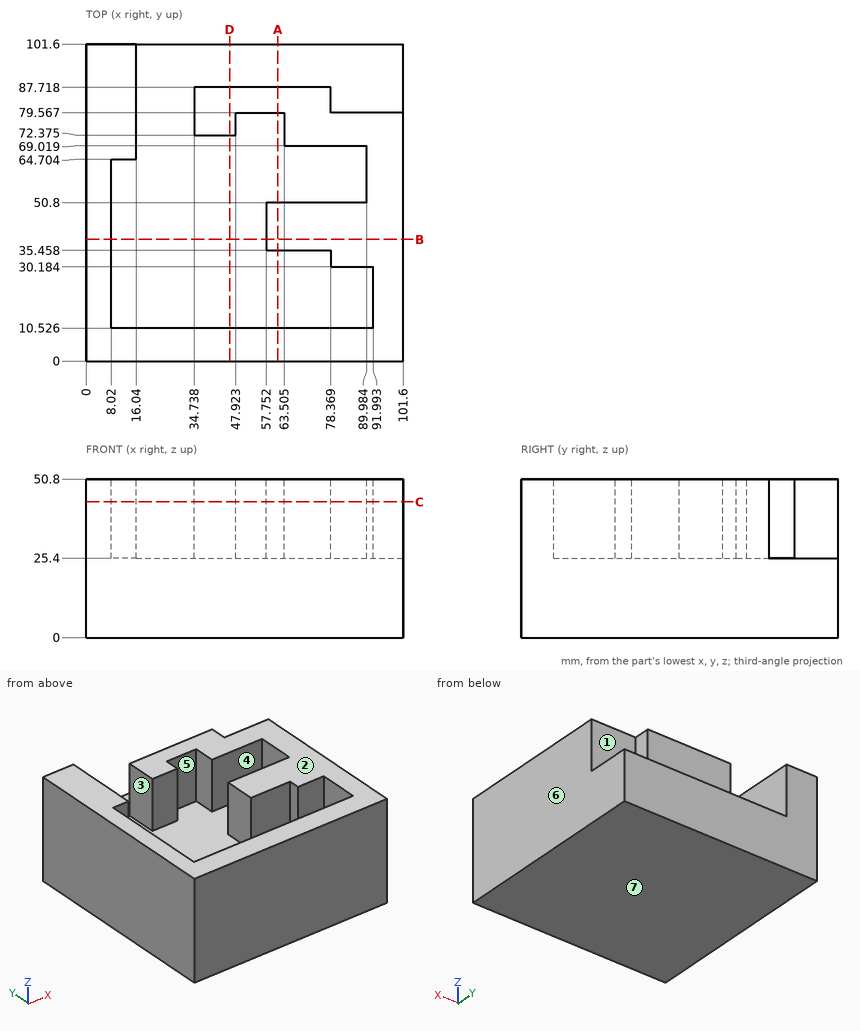
Geometry check sheet. Reference: drawing and pictorial views, mm from the part's lowest x, y, z. A direction names the side the tool comes from. Round coordinates to 2 decimals unless told otherwise and drop trailing zeros. Write each loop counter-clockwise with the first axis right and the second up, starting at its lowest first coordinate (ties: lowest second). Pieces come first, ordered by that corner, then holes.
(1) Depth check by flat-ended pin: pin 1 Ø6 at (x, y) = (20, 75.5) entering from +Z; pin 2 Ø6 at (x, z) = (85.5, 42.5) entering from +Y; pin 3 Ø6 at (x, z) = (71, 37.5) entering from +Y. Enter the tip coordinate at first touch or a pass-through.
Returned:
pin 1: stops at z = 25.4
pin 2: stops at y = 79.57
pin 3: stops at y = 87.72
(2) Section check B-B (y = 39). Enter the section's corners in (x, z).
Returned:
outline: (0, 0) - (101.6, 0) - (101.6, 50.8) - (57.75, 50.8) - (57.75, 25.4) - (8.02, 25.4) - (8.02, 50.8) - (0, 50.8) - close
(3) Material ranges on line 1 (X direction, y = 64, z = 39) (1 decimal); line 2 (Y direction, x = 42.5, z = 47.5) (1 decimal); line 3 (Y direction, x = 50.5, z = 40) (1 decimal), recorded low to high.
Returned:
line 1: x = 0 to 8, 90 to 101.6
line 2: y = 0 to 10.5, 72.4 to 87.7
line 3: y = 0 to 10.5, 79.6 to 87.7
(4) Section check A-A (x = 61.5). Enter the section's corners in (y, z) (1 decimal).
Returned:
outline: (0, 0) - (101.6, 0) - (101.6, 25.4) - (87.7, 25.4) - (87.7, 50.8) - (79.6, 50.8) - (79.6, 25.4) - (50.8, 25.4) - (50.8, 50.8) - (35.5, 50.8) - (35.5, 25.4) - (10.5, 25.4) - (10.5, 50.8) - (0, 50.8) - close
(5) Access from +Z, -Z, +X, -X, +Y, -Y to the whole of each face (thin tool, end or side, straight path). Record for the marked faces 1, 2, 3 and 4.
Returned:
face 1: +Z, +X, +Y
face 2: +Z, +X, -X, +Y, -Y
face 3: +Z, +Y
face 4: +Z
(6) Mould release check, pull along X, two halves, no side actions. Record for the marked faces 5, 6 and 7: pulls with the +X half, pulls with the -X half, needs draft (parallel to the pull), parting line crosses it, or undercut.
Returned:
face 5: undercut
face 6: pulls with the +X half
face 7: needs draft
(7) Section check D-D (x = 46). Enter the section's corners in (y, z) (1 decimal).
Returned:
outline: (0, 0) - (101.6, 0) - (101.6, 25.4) - (87.7, 25.4) - (87.7, 50.8) - (72.4, 50.8) - (72.4, 25.4) - (10.5, 25.4) - (10.5, 50.8) - (0, 50.8) - close
(8) Section check C-C (z = 43.5). Enter the section's corners in (x, y) (1 decimal), plus the area to 3 significant figures.
Returned:
outline: (0, 0) - (101.6, 0) - (101.6, 79.6) - (78.4, 79.6) - (78.4, 87.7) - (34.7, 87.7) - (34.7, 72.4) - (47.9, 72.4) - (47.9, 79.6) - (63.5, 79.6) - (63.5, 69) - (90, 69) - (90, 50.8) - (78.4, 50.8) - (57.8, 50.8) - (57.8, 35.5) - (78.4, 35.5) - (78.4, 30.2) - (92, 30.2) - (92, 10.5) - (8, 10.5) - (8, 64.7) - (16, 64.7) - (16, 101.6) - (0, 101.6) - close
area: 4,140 mm2
